Geometry check sheet. Reference: the model listing, model coordinates, mm. Round coordinates to 2 decimals unless told otherwise and drop trailing zeros. Write each loop counter-clockwise with the first axis right and the second up, starting at its lowest first coordinate (ties: lowest second). Pieces come first, ordered by that corner, then holes.
Item 1: Cross-section at A-A (y = 5.85). Enter the section's corners in (x, z), then the cut area to 3 significant figures.
Item 2: Cross-section at C-C (z = -65). Enter the section's corners in (x, y), then the cut area to 3 significant figures.
Item 3: Scan lines: probe 1 along Z at (x, y) = (-135.5, 5.8); probe 2 along X at (y, z) = (7.15, -82); probe 3 along X at (y, z) = (5.5, 66). Record each from-to range of solid material in increasing order.
Item 4: Depth check by flat-ended pin: P1, Ø4.5, axis at x = -147.83, z = 6.77, coming from the -Y side. Enter the tip coordinate at first touch or a pass-through.
Item 5: Cross-section at B-B (z = 53.5). Enter the section's corners in (x, y).
from build123d import *

# Parameters (mm, degrees)
SKETCH1_R           = 2.5527
BOSS_EXTRUDE1_DEPTH = 3.175


with BuildPart() as part:
    # Sketch1 → Boss-Extrude1 (new body)
    with BuildSketch(Plane(origin=(0, 7.659460084, 0), x_dir=(1, 0, 0), z_dir=(0, 1, 0))):
        Polygon((-141.5163305, 104.251042847), (-124.323681089, 104.251042847), (-124.323681089, -117.799669373), (-141.5163305, -117.799669373), (-157.82954988, -6.774313263), align=None)
        with Locations(Location((-136.5163305, -96.185148791, 0), (0, 0, 270))):
            Circle(SKETCH1_R, mode=Mode.SUBTRACT)
        with Locations(Location((-147.82954988, -6.774313263, 0), (0, 0, 270))):
            Circle(SKETCH1_R, mode=Mode.SUBTRACT)
        with Locations(Location((-136.5163305, 82.636522264, 0), (0, 0, 270))):
            Circle(SKETCH1_R, mode=Mode.SUBTRACT)
    extrude(amount=-BOSS_EXTRUDE1_DEPTH)


solid = part.part
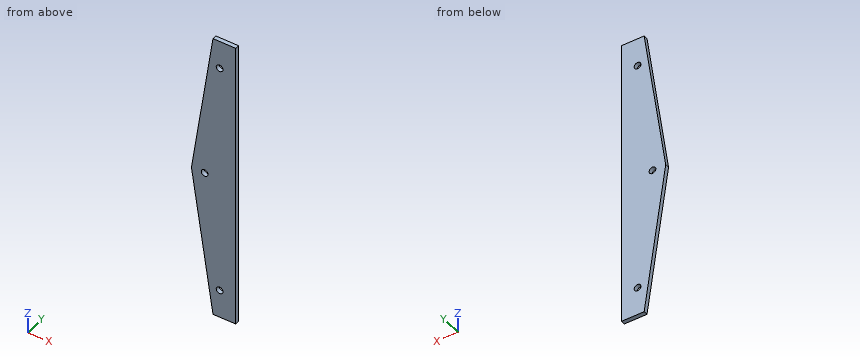
Resolved:
1. outline: (-157.83, 6.77) - (-141.52, -104.25) - (-124.32, -104.25) - (-124.32, 117.8) - (-141.52, 117.8) - close; hole circle Ø5.11 at (-147.83, 6.77); hole circle Ø5.11 at (-136.52, -82.64); hole circle Ø5.11 at (-136.52, 96.19)
1. area: 5,570 mm2
2. outline: (-147.28, 4.48) - (-124.32, 4.48) - (-124.32, 7.66) - (-147.28, 7.66) - close
2. area: 72.9 mm2
3. probe 1: z = -104.25 to -84.98, -80.29 to 93.84, 98.53 to 117.8
3. probe 2: x = -144.79 to -138.99, -134.04 to -124.32
3. probe 3: x = -149.13 to -124.32
4. P1: passes through
5. outline: (-150.96, 4.48) - (-124.32, 4.48) - (-124.32, 7.66) - (-150.96, 7.66) - close
